Check sheet for the modelled part. Datum: model origin and axes. Units: mm. Face numbers are marked on the shaded views. A direction names the side the tool comes from. Coordinates: 2 decimals unless noted, no trailing zeros. Loops run counter-clockwise (first coordinate to the right, second up) from the corner with the lowest first, then second, coordinate; pieces in that order, holes last. Notation, with made-up numbers: (37, 75) -> (41, 75) arc R18 ccw to (41, 81) -> close; hole circle Ø7 at (12.5, 83). An arc over 180 degrees is marked (long way). Use CSV: the item, a comma, the result in double quotes.
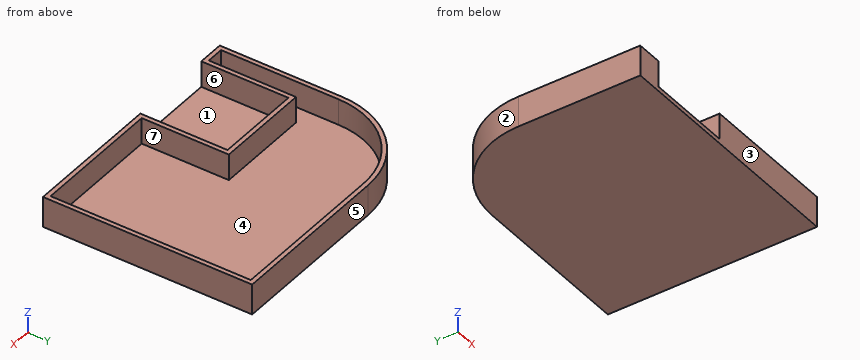
```python
from build123d import *

# Parameters (mm, degrees)
F1_DEPTH = 3.2512
F3_DEPTH = 19.05


with BuildPart() as f1:
    # F0 (on Top) → F1 (new body)
    with BuildSketch(Plane.XY):
        with BuildLine():
            Line((92.075, 76.2), (-28.575, 76.2))
            ThreePointArc((-28.575, 76.2), (-73.476281, 57.601281), (-92.075, 12.7))
            Line((-92.075, 12.7), (-92.075, -76.2))
            Line((-92.075, -76.2), (92.075, -76.2))
            Line((92.075, -76.2), (92.075, 76.2))
        make_face()
    extrude(amount=F1_DEPTH)

    # F2 (on face) → F3 (join)
    with BuildSketch(Plane.XY.offset(3.2512)):
        with BuildLine():
            Line((-72.8726, -76.2), (-72.8726, -12.7))
            Line((-72.8726, -12.7), (-9.3726, -12.7))
            Line((-9.3726, -12.7), (-9.3726, -76.2))
            Line((-9.3726, -76.2), (92.075, -76.2))
            Line((92.075, -76.2), (92.075, 76.2))
            Line((92.075, 76.2), (-28.575, 76.2))
            ThreePointArc((-28.575, 76.2), (-73.476281, 57.601281), (-92.075, 12.7))
            Line((-92.075, 12.7), (-92.075, -76.2))
            Line((-92.075, -76.2), (-72.8726, -76.2))
        make_face()
        with BuildLine():
            Line((-28.575, 72.9488), (88.8238, 72.9488))
            Line((88.8238, 72.9488), (88.8238, -72.9488))
            Line((88.8238, -72.9488), (-6.1214, -72.9488))
            Line((-6.1214, -72.9488), (-6.1214, -9.4488))
            Line((-6.1214, -9.4488), (-76.1238, -9.4488))
            Line((-76.1238, -9.4488), (-76.1238, -72.9488))
            Line((-76.1238, -72.9488), (-88.8238, -72.9488))
            Line((-88.8238, -72.9488), (-88.8238, 12.7))
            ThreePointArc((-88.8238, 12.7), (-71.177335, 55.302335), (-28.575, 72.9488))
        make_face(mode=Mode.SUBTRACT)
    extrude(amount=F3_DEPTH)


solid = f1.part
```
1) Draft check along Y on the marked faces 1, 2, 3 and 4. Enter one of: released by +Y, released by -Y, zero draft, split by the parting line, or undercut.
Answer below:
face 1,"zero draft"
face 2,"released by +Y"
face 3,"released by -Y"
face 4,"undercut"
2) Cross-section at C-C on y = -42.5. Record the boundary of the cut face in (x, z) (3 decimals).
Answer below:
outline,"(-92.075, 0) -> (92.075, 0) -> (92.075, 22.301) -> (88.824, 22.301) -> (88.824, 3.251) -> (-6.121, 3.251) -> (-6.121, 22.301) -> (-9.373, 22.301) -> (-9.373, 3.251) -> (-72.873, 3.251) -> (-72.873, 22.301) -> (-76.124, 22.301) -> (-76.124, 3.251) -> (-88.824, 3.251) -> (-88.824, 22.301) -> (-92.075, 22.301) -> close"
3) Access from +Z, -Z, +X, -X, +Y, -Y to the whole of each face (thin tool, end or side, straight path). Record for the marked faces 5, 6 and 7.
Answer below:
face 5,"+Z, -Z, +X, -X, +Y"
face 6,"+Z, -Y"
face 7,"+Z"
4) Thickness scan on line 1 along X through (y, z) = (-33, 13) (3 decimals); line 2 along Y through (x, z) = (13.5, 3.75); line 3 along X through (y, z) = (-9.5, 20) (3 decimals). Record the ranges inside material, lowest first. Write a range as from..to.
Answer below:
line 1,"x = -92.075..-88.824, -76.124..-72.873, -9.373..-6.121, 88.824..92.075"
line 2,"y = -76.2..-72.95, 72.95..76.2"
line 3,"x = -92.075..-88.824, -76.124..-6.121, 88.824..92.075"
5) Cross-section at A-A on z = 13.75. Record the boundary of the cut face in (x, y) (3 decimals), and give its area (3 significant figures).
Answer below:
outline,"(-92.075, -76.2) -> (-72.873, -76.2) -> (-72.873, -12.7) -> (-9.373, -12.7) -> (-9.373, -76.2) -> (92.075, -76.2) -> (92.075, 76.2) -> (-28.575, 76.2) arc R63.5 ccw to (-92.075, 12.7) -> close; hole (-88.824, -72.949) -> (-76.124, -72.949) -> (-76.124, -9.449) -> (-6.121, -9.449) -> (-6.121, -72.949) -> (88.824, -72.949) -> (88.824, 72.949) -> (-28.575, 72.949) arc R60.249 ccw to (-88.824, 12.7) -> close"
area,"2,470 mm²"
6) Cross-section at D-D on y = 32.5. Record the boundary of the cut face in (x, z) (3 decimals), and give its area (3 significant figures).
Answer below:
outline,"(-88.909, 0) -> (92.075, 0) -> (92.075, 22.301) -> (88.824, 22.301) -> (88.824, 3.251) -> (-85.477, 3.251) -> (-85.477, 22.301) -> (-88.909, 22.301) -> close"
area,"716 mm²"
7) Cross-section at B-B on x = -25. Record the boundary of the cut face in (y, z), and give its area (3 significant figures).
Answer below:
outline,"(-76.2, 0) -> (76.2, 0) -> (76.2, 22.3) -> (72.95, 22.3) -> (72.95, 3.25) -> (-9.45, 3.25) -> (-9.45, 22.3) -> (-12.7, 22.3) -> (-12.7, 3.25) -> (-76.2, 3.25) -> close"
area,"619 mm²"
8) Go/stop test with flat-tipped pins: pin 1 Ø6 at (x, z) = (-70.5, 18) entering from +Y; pin 2 Ø10 at (x, z) = (-68, 7) entering from +Y; pin 3 Ø9.5 at (x, z) = (-33.5, 11.5) entering from -Y. Record where each tip stops, or that it passes through.
Answer below:
pin 1,"stops at y = 62.87"
pin 2,"stops at y = 66.06"
pin 3,"stops at y = -12.7"
